Source: CAD feature listing. Evaluate the final solid. Frame: model axes, mm. Face numbers are marked on the shaded views. A direction names the side the tool comes from. Give positions to 0.01 mm unless a question says otherwise; leave off trailing zeros. Write each loop counter-clockwise with the first axis right and the second up, starting at its lowest first coordinate (ties: lowest second). Pieces come first, ordered by that corner, then holes.
```python
from build123d import *

# Parameters (mm, degrees)
F0_R     = 6.75
F0_R_2   = 11
F1_DEPTH = 7


with BuildPart() as f1:
    # F0 (on Top) → F1 (new body)
    with BuildSketch(Plane.XY):
        with BuildLine():
            Line((12.750323, 51.767008), (-12.814607, 51.767008))
            ThreePointArc((-12.814607, 51.767008), (-17.304735, 49.907136), (-19.164607, 45.417008))
            Line((-19.164607, 45.417008), (-19.164607, -43.482992))
            ThreePointArc((-19.164607, -43.482992), (-17.304735, -47.97312), (-12.814607, -49.832992))
            Line((-12.814607, -49.832992), (12.750323, -49.832992))
            ThreePointArc((12.750323, -49.832992), (17.240451, -47.97312), (19.100323, -43.482992))
            Line((19.100323, -43.482992), (19.100323, 45.417008))
            ThreePointArc((19.100323, 45.417008), (17.240451, 49.907136), (12.750323, 51.767008))
        make_face()
        Polygon((7.505553, -37), (3.752777, -43.5), (-3.752777, -43.5), (-7.505553, -37), (-3.752777, -30.5), (3.752777, -30.5), align=None, mode=Mode.SUBTRACT)
        with Locations((0, -20.269467)):
            Circle(F0_R, mode=Mode.SUBTRACT)
        Circle(F0_R_2, mode=Mode.SUBTRACT)
        with Locations((0, 20.228889)):
            Circle(F0_R, mode=Mode.SUBTRACT)
        Polygon((1.442276, 44.365675), (7.1, 39.43379), (5.657724, 32.068115), (-1.442276, 29.634325), (-7.1, 34.56621), (-5.657724, 41.931885), align=None, mode=Mode.SUBTRACT)
    extrude(amount=F1_DEPTH)


solid = f1.part
```
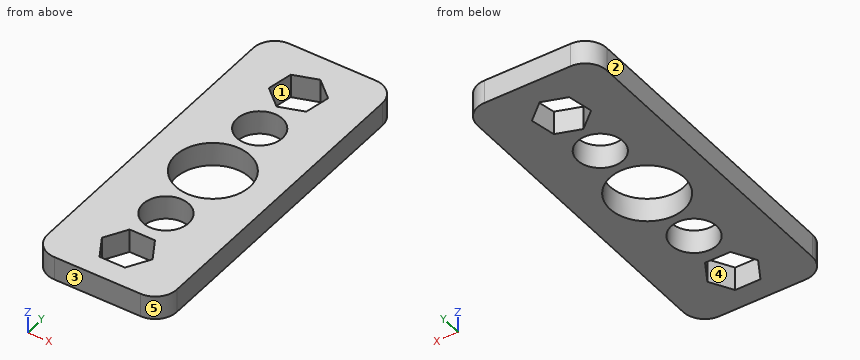
1. Section query C-C (z = 3.25). Return loops of the section in (x, y), plus the area to 3 significant figures.
2. Pin query (flat end, axial travel): P1, Ø17.5, axis at x = 0, y = 0, coming from the +Z side. Return the tip coordinate at first contact, or that it passes through.
3. Section query D-D (x = 9). Return loops of the section in (y, z), plus the area to 3 significant figures.
4. Section query A-A (y = 0). Return loops of the section in (x, z).
5. Pull-direction query (X, two-part tool) for the marked faces 1, 2 and 3; classes: pulls with the +X half, pulls with the -X half, needs draft (parallel to the pull), parting line crosses it, or undercut.
6. Access query for the marked faces 4 and 5. Directions: +Z, -Z, +X, -X, +Y, -Y. A direction counts if a zero-diameter tool reaches every point of the face in a straight line with its end or side. Return the directions, or none.
7. Line query: probe 1 along Y at (x, z) = (0, 5); probe 2 along Y at (x, z) = (9, 2.5); probe 3 along X at (y, z) = (-42.5, 4). Output: solid intervals per line, ascending.
8. Section query B-B (x = 0). Return loops of the section in (y, z), plus the area to 3 significant figures.
The answers:
1. outline: (-19.16, -43.48) arc R6.35 ccw to (-12.81, -49.83) - (12.75, -49.83) arc R6.35 ccw to (19.1, -43.48) - (19.1, 45.42) arc R6.35 ccw to (12.75, 51.77) - (-12.81, 51.77) arc R6.35 ccw to (-19.16, 45.42) - close; hole circle Ø22 at (0, 0); hole (-7.51, -37) - (-3.75, -43.5) - (3.75, -43.5) - (7.51, -37) - (3.75, -30.5) - (-3.75, -30.5) - close; hole (-7.1, 34.57) - (-1.44, 29.63) - (5.66, 32.07) - (7.1, 39.43) - (1.44, 44.37) - (-5.66, 41.93) - close; hole circle Ø13.5 at (0, -20.27); hole circle Ø13.5 at (0, 20.23)
1. area: 2,890 mm2
2. P1: passes through
3. outline: (-49.83, 0) - (-6.32, 0) - (-6.32, 7) - (-49.83, 7) - close; (6.32, 0) - (51.77, 0) - (51.77, 7) - (6.32, 7) - close
3. area: 623 mm2
4. outline: (-19.16, 0) - (-11, 0) - (-11, 7) - (-19.16, 7) - close; (11, 0) - (19.1, 0) - (19.1, 7) - (11, 7) - close
5. face 1: undercut
5. face 2: pulls with the -X half
5. face 3: needs draft
6. face 4: +Z, -Z
6. face 5: +Z, -Z, +X, -Y
7. probe 1: y = -49.83 to -43.5, -30.5 to -27.02, -13.52 to -11, 11 to 13.48, 26.98 to 30.13, 43.87 to 51.77
7. probe 2: y = -49.83 to -6.32, 6.32 to 51.77
7. probe 3: x = -19.16 to -4.33, 4.33 to 19.1
8. outline: (-49.83, 0) - (-43.5, 0) - (-43.5, 7) - (-49.83, 7) - close; (-30.5, 0) - (-27.02, 0) - (-27.02, 7) - (-30.5, 7) - close; (-13.52, 0) - (-11, 0) - (-11, 7) - (-13.52, 7) - close; (11, 0) - (13.48, 0) - (13.48, 7) - (11, 7) - close; (26.98, 0) - (30.13, 0) - (30.13, 7) - (26.98, 7) - close; (43.87, 0) - (51.77, 0) - (51.77, 7) - (43.87, 7) - close
8. area: 181 mm2
